Check sheet for the modelled part. Datum: model origin and axes. Units: mm. A direction names the side the tool comes from. Give positions to 0.01 mm unless a question says otherwise; leave off trailing zeros. Order: outer loops, then holes, each group sorted by start corner. A loop starts at its lowest first (then second) coordinate and runs counter-clockwise, first axis right, second up.
```python
from build123d import *

# Parameters (mm, degrees)
BOSS_EXTRUDE1_DEPTH = 100
CUT_EXTRUDE5_DEPTH  = 16
CUT_EXTRUDE6_DEPTH  = 16
SKETCH8_R           = 2.415
CUT_EXTRUDE7_DEPTH  = 16
SKETCH6_R           = 2.415
CUT_EXTRUDE8_DEPTH  = 16


with BuildPart() as part:
    # Sketch1 → Boss-Extrude1 (new body)
    with BuildSketch(Plane(origin=(0, 0, 0), x_dir=(1, 0, 0), z_dir=(0, 1, 0))):
        Polygon((0, 0), (0, 13.85), (12.34, 13.85), (12.34, 11.35), (2.5, 11.35), (2.5, 0), align=None)
    extrude(amount=BOSS_EXTRUDE1_DEPTH)

    # Sketch5 → Cut-Extrude5 (cut)
    with BuildSketch(Plane(origin=(0, 0, -13.85), x_dir=(-1, 0, 0), z_dir=(0, 0, -1))):
        Polygon((0, 98.157512876), (-15.02502343, 99.39968578), (-15.02502343, 94.867790228), align=None)
    extrude(amount=-CUT_EXTRUDE5_DEPTH, mode=Mode.SUBTRACT)


with BuildPart() as body_2:
    # of the pieces the cut leaves, the one that is kept (cut_extrude5_keep)
    add(part.part.solids().sort_by_distance((0, 0, 0))[0])

    # Sketch4 → Cut-Extrude6 (cut)
    with BuildSketch(Plane.ZY):
        Polygon((-13.849977668, 98.157512876), (8.264271821, 91.866448074), (8.264271821, 98.157512876), align=None)
    extrude(amount=-CUT_EXTRUDE6_DEPTH, mode=Mode.SUBTRACT)

    # Sketch8 → Cut-Extrude7 (cut)
    with BuildSketch(Plane(origin=(2.5, 0, 0), x_dir=(0, 0, -1), z_dir=(1, 0, 0))):
        with Locations((5.675, 35)):
            Circle(SKETCH8_R)
        with Locations((5.675, 60.83189408)):
            Circle(SKETCH8_R)
    extrude(amount=-CUT_EXTRUDE7_DEPTH, mode=Mode.SUBTRACT)

    # Sketch6 → Cut-Extrude8 (cut)
    with BuildSketch(Plane.XY.offset(-11.35)):
        with Locations((7.42, 20)):
            Circle(SKETCH6_R)
        with Locations((7.42, 76.450996936)):
            Circle(SKETCH6_R)
    extrude(amount=-CUT_EXTRUDE8_DEPTH, mode=Mode.SUBTRACT)


solid = body_2.part
```
(1) Sectioned sample at B-B (x = 8.25). Enter the section's corners in (y, z), plus the area to 3 significant figures.
(2) Sectioned sample at C-C (z = -12.75). Enter the section's corners in (x, y) (3 decimals), plus the area to 3 significant figures.
(3) Thickness scan on L1, parallel to Z at x = 5, y = 92.5; L2, parallel to X at y = 50.5, z = -6; L3, parallel to Y at x = 7.42, z = -12 (3 decimals). Record the ranges inside material, lowest first.
(4) Sectioned sample at D-D (z = -4.5). Enter the section's corners in (x, y), plus the area to 3 significant figures.
(5) Tool access check on faces 4 (the face through (12.34, 47, -13)), 5 (the face through (7, 48, -11.35)). Record the directions out of +Z, -Z, +X, -X, +Y, -Y that give a thin tool (end or side, any length) a straight path to the whole face; none if there is none.
(6) Sectioned sample at A-A (y = 35). Enter the section's corners in (x, z), plus the area to 4 significant figures.
(7) Go/stop test with flat-tipped pins: P1, Ø5, axis at x = 8, y = 64.5, coming from the +Z side; P2, Ø8, axis at y = 75, z = -6, coming from the +X side. Record where each tip stops, or that it passes through.
(8) Release check for a two-part mould opening along X. For faces 1 (the face through (8.534, 17.857, -12.582)), 2 (the face through (1.268, 58.474, -5.151)), 3 (the face through (7.627, 96.487, -12.617)) record: released by +X, released by -X, zero draft, split by the parting line, or undercut.
Values follow:
1. outline: (0, -13.85) - (17.73, -13.85) - (17.73, -11.35) - (0, -11.35) - close; (22.27, -13.85) - (74.18, -13.85) - (74.18, -11.35) - (22.27, -11.35) - close; (78.72, -13.85) - (96.35, -13.85) - (96.35, -11.35) - (78.72, -11.35) - close
1. area: 218 mm2
2. outline: (0, 0) - (12.34, 0) - (12.34, 95.456) - (1.429, 97.845) - (0, 97.845) - close; hole circle Ø4.83 at (7.42, 20); hole circle Ø4.83 at (7.42, 76.451)
2. area: 1,160 mm2
3. L1: z = -13.85 to -11.35
3. L2: x = 0 to 2.5
3. L3: y = 0 to 17.585, 22.415 to 74.036, 78.866 to 96.533
4. outline: (0, 0) - (2.5, 0) - (2.5, 32.89) - (0, 32.89) - close; (0, 37.11) - (2.5, 37.11) - (2.5, 58.72) - (0, 58.72) - close; (0, 62.94) - (2.5, 62.94) - (2.5, 95.5) - (0, 95.5) - close
4. area: 218 mm2
5. face 4: +Z, -Z, +X, +Y, -Y
5. face 5: +Z, +X, +Y, -Y
6. outline: (0, -13.85) - (12.34, -13.85) - (12.34, -11.35) - (2.5, -11.35) - (2.5, -8.09) - (0, -8.09) - close; (0, -3.26) - (2.5, -3.26) - (2.5, 0) - (0, 0) - close
6. area: 47.15 mm2
7. P1: stops at z = -11.35
7. P2: stops at x = 2.5
8. face 1: undercut
8. face 2: zero draft
8. face 3: released by +X
